from build123d import *

# Parameters (mm, degrees)
SKETCH2_R           = 0.4
BOSS_EXTRUDE1_DEPTH = 18
CUT_EXTRUDE1_DEPTH  = 17


with BuildPart() as part:
    # Sketch2 → Boss-Extrude1 (new body)
    with BuildSketch(Plane(origin=(0, 0, 0), x_dir=(1, 0, 0), z_dir=(0, 1, 0))):
        with BuildLine():
            Line((-20, 9.723165676), (-20, -9.723165676))
            ThreePointArc((-20, -9.723165676), (-19.186684057, -11.686684057), (-17.223165676, -12.5))
            Line((-17.223165676, -12.5), (17.223165676, -12.5))
            ThreePointArc((17.223165676, -12.5), (19.186684057, -11.686684057), (20, -9.723165676))
            Line((20, -9.723165676), (20, 9.723165676))
            ThreePointArc((20, 9.723165676), (19.186684057, 11.686684057), (17.223165676, 12.5))
            Line((17.223165676, 12.5), (-17.223165676, 12.5))
            ThreePointArc((-17.223165676, 12.5), (-19.186684057, 11.686684057), (-20, 9.723165676))
        make_face()
        with Locations(Location((0, 0, 0), (0, 0, 270))):
            Circle(SKETCH2_R, mode=Mode.SUBTRACT)
    extrude(amount=BOSS_EXTRUDE1_DEPTH)

    # Sketch3 → Cut-Extrude1 (cut)
    with BuildSketch(Plane.XZ):
        with BuildLine():
            Line((19, -9.723165676), (19, 9.723165676))
            ThreePointArc((19, 9.723165676), (18.479577276, 10.979577276), (17.223165676, 11.5))
            Line((17.223165676, 11.5), (-17.223165676, 11.5))
            ThreePointArc((-17.223165676, 11.5), (-18.479577276, 10.979577276), (-19, 9.723165676))
            Line((-19, 9.723165676), (-19, -9.723165676))
            ThreePointArc((-19, -9.723165676), (-18.479577276, -10.979577276), (-17.223165676, -11.5))
            Line((-17.223165676, -11.5), (17.223165676, -11.5))
            ThreePointArc((17.223165676, -11.5), (18.479577276, -10.979577276), (19, -9.723165676))
        make_face()
    extrude(amount=-CUT_EXTRUDE1_DEPTH, mode=Mode.SUBTRACT)


solid = part.part
Geometry: final body of the model. Coordinates: model frame, mm. A direction names the side the tool comes from. Give positions to 0.01 mm unless a question says otherwise; leave off trailing zeros. Write each loop counter-clockwise with the first axis right and the second up, starting at its lowest first coordinate (ties: lowest second). Pieces come first, ordered by that corner, then holes. Notation, with made-up numbers: (-18, 73.25) -> (34, 73.25) arc R22 ccw to (34, 109.25) -> close; hole circle Ø4 at (8, 24.5). An arc over 180 degrees is marked (long way). Answer as a JSON object with one key per item and string values.
1. Cut plane A-A on y = 4.25. Output: boundary loops of the cut face in (x, z).
Ans:
{"outline": "(-20, -9.72) arc R2.78 ccw to (-17.22, -12.5) -> (17.22, -12.5) arc R2.78 ccw to (20, -9.72) -> (20, 9.72) arc R2.78 ccw to (17.22, 12.5) -> (-17.22, 12.5) arc R2.78 ccw to (-20, 9.72) -> close; hole (-19, -9.72) arc R1.78 ccw to (-17.22, -11.5) -> (17.22, -11.5) arc R1.78 ccw to (19, -9.72) -> (19, 9.72) arc R1.78 ccw to (17.22, 11.5) -> (-17.22, 11.5) arc R1.78 ccw to (-19, 9.72) -> close"}
2. Ray query, probe 1 along Z at (x, y) = (16, 15); probe 2 along Z at (x, y) = (0, 17.3); probe 3 along X at (y, z) = (14, -0.75). Return the intervals inside material, ascending. Write a range as from..to.
Ans:
{"probe 1": "z = -12.5..-11.5, 11.5..12.5", "probe 2": "z = -12.5..-0.4, 0.4..12.5", "probe 3": "x = -20..-19, 19..20"}
3. Cut plane C-C on z = 3. Output: boundary loops of the cut face in (x, y), and give its area (3 significant figures).
Ans:
{"outline": "(-20, 0) -> (-19, 0) -> (-19, 17) -> (19, 17) -> (19, 0) -> (20, 0) -> (20, 18) -> (-20, 18) -> close", "area": "74.0 mm^2"}
4. Access query for faces 1 (the cylindrical face through (-19.165, 8.874, -11.708)), 2 (the cylindrical face through (18.47, 8.38, -10.99)). Directions: +Z, -Z, +X, -X, +Y, -Y. A direction counts if a zero-diameter tool reaches every point of the face in a straight line with its end or side. Return the directions, or none.
Ans:
{"face 1": "-Z, -X, +Y, -Y", "face 2": "-Y"}
5. Mould query, pull axis Z, two halves, no side actions, for faces 3 (the cylindrical face through (-19.208, 8.874, 11.665)), 4 (the flat face through (0, 18, -3)), 5 (the cylindrical face through (-18.47, 8.38, 10.99)). Classes: pulls with the +Z half, pulls with the -Z half, needs draft (parallel to the pull), parting line crosses it, or undercut.
Ans:
{"face 3": "pulls with the +Z half", "face 4": "needs draft", "face 5": "undercut"}
6. Cut plane B-B on x = 1.5. Output: boundary loops of the cut face in (y, z).
Ans:
{"outline": "(0, -12.5) -> (18, -12.5) -> (18, 12.5) -> (0, 12.5) -> (0, 11.5) -> (17, 11.5) -> (17, -11.5) -> (0, -11.5) -> close"}
